Source: CAD feature listing. Evaluate the final solid. Frame: model axes, mm. Face numbers are marked on the shaded views. Round coordinates to 2 decimals unless told otherwise and drop trailing zeros. Write each loop counter-clockwise with the first axis right and the second up, starting at its lowest first coordinate (ties: lowest second). Pieces come first, ordered by that corner, then holes. Notation, with made-up numbers: M -25.5,-37.75 L 16.5,-37.75 A34 cw 16.5,-2.75 Z; hole C 0.5,52.5 d11. An arc over 180 degrees is marked long. Answer in a Markdown table with one row per item. Add a question column.
Item 1: Mould query, pull axis Y, two halves, no side actions, for the marked faces 1, 2 and 3. Classes: released by +Y, released by -Y, zero draft, split by the parting line, or undercut.
Item 2: Material intervals for probe 1 along Z at (x, y) = (38, 22.5); probe 2 along Y at (x, z) = (0, 31); probe 3 along Y at (x, z) = (0, 12), sorted ascending.
Item 3: Cut plane A-A on z = 39.5. Return loops of the section in (x, y), and give its area (3 significant figures).
Item 4: Contact query for flat-ended pins moving along their axis: pin 1 (4 mm diameter, centred on y = 6.5, z = 36.5, fed in from -X); pin 2 (2 mm diameter, centred on y = 1, z = 41.5, fed in from +X); pin 3 (4 mm diameter, centred on x = -6, z = 6, fed in from -Y). Output: stop coordinate, or through.
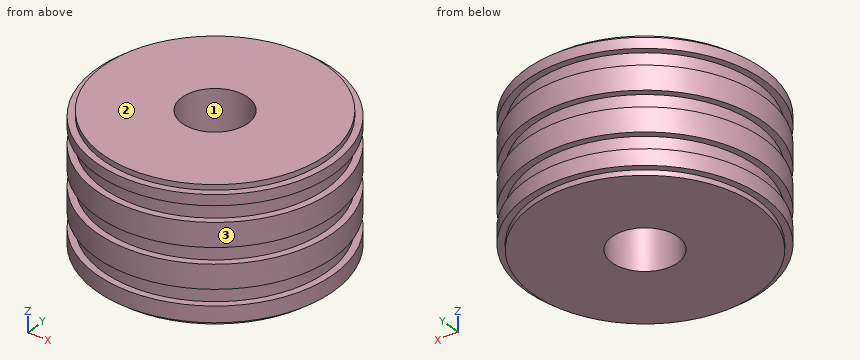
from build123d import *

# Parameters (mm, degrees)
SKETCH_1_R             = 45
EXTRUDE_1_DEPTH        = 50
CUT_EXTRUDE_START      = -6
SKETCH_2_R             = 45
SKETCH_2_R_2           = 42.5
CUT_EXTRUDE_1_DEPTH    = 6
PATTERN_LINEAR_1_COUNT = 3
PATTERN_LINEAR_1_PITCH = 15
SKETCH_3_R             = 45
SKETCH_3_R_2           = 42.5
CUT_EXTRUDE_2_DEPTH    = 2
SKETCH_4_R             = 45
SKETCH_4_R_2           = 42.5
CUT_EXTRUDE_4_DEPTH    = 2
SKETCH_5_R             = 12.5
CUT_EXTRUDE_5_DEPTH    = 51


with BuildPart() as part:
    # 草图1 → 凸台-拉伸1 (new body)
    with BuildSketch(Plane.XY):
        Circle(SKETCH_1_R)
    extrude(amount=EXTRUDE_1_DEPTH)

    # 草图2 → 切除-拉伸1 (cut)
    with BuildSketch(Plane.XY.offset(50).offset(CUT_EXTRUDE_START)):
        Circle(SKETCH_2_R)
        Circle(SKETCH_2_R_2, mode=Mode.SUBTRACT)
    cut_extrude_1 = extrude(amount=-CUT_EXTRUDE_1_DEPTH, mode=Mode.SUBTRACT)

    # 阵列(线性)1: 切除-拉伸1 ×3
    with Locations(*[(0, 0, -i * PATTERN_LINEAR_1_PITCH) for i in range(1, PATTERN_LINEAR_1_COUNT)]):
        add(cut_extrude_1, mode=Mode.SUBTRACT)

    # 草图3 → 切除-拉伸2 (cut)
    with BuildSketch(Plane.XY.offset(50)):
        Circle(SKETCH_3_R)
        Circle(SKETCH_3_R_2, mode=Mode.SUBTRACT)
    extrude(amount=-CUT_EXTRUDE_2_DEPTH, mode=Mode.SUBTRACT)

    # 草图4 → 切除-拉伸4 (cut)
    with BuildSketch(Plane(origin=(0, 0, 0), x_dir=(-1, 0, 0), z_dir=(0, 0, -1))):
        Circle(SKETCH_4_R)
        Circle(SKETCH_4_R_2, mode=Mode.SUBTRACT)
    extrude(amount=-CUT_EXTRUDE_4_DEPTH, mode=Mode.SUBTRACT)

    # 草图5 → 切除-拉伸5 (cut, through all)
    with BuildSketch(Plane(origin=(0, 0, 0), x_dir=(-1, 0, 0), z_dir=(0, 0, -1))):
        Circle(SKETCH_5_R)
    extrude(amount=-CUT_EXTRUDE_5_DEPTH, mode=Mode.SUBTRACT)


solid = part.part
Results below:
| question | item | result |
|---|---|---|
| 1 | face 1 | undercut |
| 1 | face 2 | zero draft |
| 1 | face 3 | split by the parting line |
| 2 | probe 1 | 2 to 8, 14 to 23, 29 to 38, 44 to 48 |
| 2 | probe 2 | -45 to -12.5, 12.5 to 45 |
| 2 | probe 3 | -42.5 to -12.5, 12.5 to 42.5 |
| 3 | outline | C 0,0 d85; hole C 0,0 d25 |
| 3 | area | 5,180 mm2 |
| 4 | pin 1 | x = -44.77 |
| 4 | pin 2 | x = 42.5 |
| 4 | pin 3 | y = -44.82 |
